```python
from build123d import *

# Parameters (mm, degrees)
SKETCH1_W                = 48
SKETCH1_H                = 20
BOSS_EXTRUDE1_DEPTH      = 300
BOSS_EXTRUDE2_DEPTH      = 24
BOSS_EXTRUDE2_DEPTH_BACK = 24
SKETCH2_R                = 20
BOSS_EXTRUDE3_DEPTH      = 24
BOSS_EXTRUDE3_DEPTH_BACK = 24
SKETCH3_R                = 20
CUT_EXTRUDE1_DEPTH       = 50
CUT_EXTRUDE1_DEPTH_BACK  = 50
SKETCH4_R                = 10
CUT_EXTRUDE2_DEPTH       = 50
CUT_EXTRUDE2_DEPTH_BACK  = 50
SKETCH5_R                = 10


with BuildPart() as part:
    # Sketch1 → Boss-Extrude1 (new body)
    with BuildSketch(Plane(origin=(0, 0, 0), x_dir=(0, 0, -1), z_dir=(1, 0, 0))):
        Rectangle(SKETCH1_W, SKETCH1_H)
    extrude(amount=BOSS_EXTRUDE1_DEPTH)

    # Sketch2 → Boss-Extrude2 (add, two sides: drawn at the far end of the back side and taken through both)
    with BuildSketch(Plane(origin=(0, 0, 0), x_dir=(1, 0, 0), z_dir=(0, 1, 0)).offset(-BOSS_EXTRUDE2_DEPTH_BACK)):
        with Locations(Location((0, 0, 0), (0, 0, 270))):
            Circle(SKETCH2_R)
    extrude(amount=BOSS_EXTRUDE2_DEPTH + BOSS_EXTRUDE2_DEPTH_BACK)

    # Sketch3 → Boss-Extrude3 (add, two sides: drawn at the far end of the back side and taken through both)
    with BuildSketch(Plane(origin=(0, 0, 0), x_dir=(1, 0, 0), z_dir=(0, 1, 0)).offset(-BOSS_EXTRUDE3_DEPTH_BACK)):
        with Locations(Location((300, 0, 0), (0, 0, 270))):
            Circle(SKETCH3_R)
    extrude(amount=BOSS_EXTRUDE3_DEPTH + BOSS_EXTRUDE3_DEPTH_BACK)

    # Sketch4 → Cut-Extrude1 (cut, two sides: drawn at the far end of the back side and taken through both)
    with BuildSketch(Plane(origin=(0, 0, 0), x_dir=(1, 0, 0), z_dir=(0, 1, 0)).offset(-CUT_EXTRUDE1_DEPTH_BACK)):
        with Locations(Location((0, 0, 0), (0, 0, 270))):
            Circle(SKETCH4_R)
    extrude(amount=CUT_EXTRUDE1_DEPTH + CUT_EXTRUDE1_DEPTH_BACK, mode=Mode.SUBTRACT)

    # Sketch5 → Cut-Extrude2 (cut, two sides: drawn at the far end of the back side and taken through both)
    with BuildSketch(Plane(origin=(0, 0, 0), x_dir=(1, 0, 0), z_dir=(0, 1, 0)).offset(-CUT_EXTRUDE2_DEPTH_BACK)):
        with Locations(Location((300, 0, 0), (0, 0, 270))):
            Circle(SKETCH5_R)
    extrude(amount=CUT_EXTRUDE2_DEPTH + CUT_EXTRUDE2_DEPTH_BACK, mode=Mode.SUBTRACT)


solid = part.part
```
CAD build for the part. Positions are in the model's coordinates, mm. A direction names the side the tool comes from. Give positions to 0.01 mm unless a question says otherwise; leave off trailing zeros. Loops run counter-clockwise (first coordinate to the right, second up) from the corner with the lowest first, then second, coordinate; pieces in that order, holes last. Notation, with made-up numbers: M 69,-33.5 L 111,-33.5 A25 cw 111,-5.5 Z; hole C -30.5,-31.5 d8. An arc over 180 degrees is marked long. Use one line per item in the form item = value.
Item 1: Which spindle directions (+Z, -Z, +X, -X, +Y, -Y) get a long thin tool onto all of the face, cutting with end or side? Do faces 4 (the face through (291.128, -0.336, 4.614)), 5 (the face through (319.83, -0.34, -2.6)). Say none if no direction does.
Determined:
face_4 = +Y, -Y
face_5 = none
Item 2: Two-plate mould, pull along X, no slides. Class faces 1 (the face through (148, -10, 0)), 2 (the face through (-19.524, -0.336, -4.336)), 3 (the face through (148, 0, -24)): pulls with the +X half, pulls with the -X half, needs draft (parallel to the pull), parting line crosses it, or undercut.
Determined:
face_1 = undercut
face_2 = undercut
face_3 = needs draft
Item 3: Drill centre lines: probe 1 along X at (y, z) = (2, 0); probe 2 along X at (y, z) = (14, 0); probe 3 along X at (y, z) = (8, -8). Where is each one in solid material? Low to high. Write a range as from..to.
Determined:
probe_1 = -20..-10, 10..290, 310..320
probe_2 = -20..-10, 10..20, 280..290, 310..320
probe_3 = -18.33..-6, 6..294, 306..318.33
Item 4: Flat gauge pins, fed straight in: pin 1 (12 mm diameter, centred on x = 96.5, z = -5.5, fed in from +Y); pin 2 (4.5 mm diameter, centred on y = 4.5, z = 22.5, fed in from -X); pin 3 (24 mm diameter, centred on x = 92, z = 7, fed in from -Y); pin 4 (12 mm diameter, centred on x = 300, z = 0, fed in from -Y). Where does each tip first touch, or does it go through?
Determined:
pin_1 = 10
pin_2 = 0
pin_3 = -10
pin_4 = through
Item 5: Slice it at D-D (x = 204). List the corners of the cut face in (y, z), plus the area to 3 significant figures.
Determined:
outline = M -10,-24 L 10,-24 L 10,24 L -10,24 Z
area = 960 mm2
Item 6: Slice it at B-B (z = 0). List the corners of the cut face in (x, y).
Determined:
outline = M -20,-24 L -10,-24 L -10,24 L -20,24 Z; M 10,-24 L 20,-24 L 20,-10 L 280,-10 L 280,-24 L 290,-24 L 290,24 L 280,24 L 280,10 L 20,10 L 20,24 L 10,24 Z; M 310,-24 L 320,-24 L 320,24 L 310,24 Z
Item 7: Slice it at A-A (y = -1). List the corners of the cut face in (x, z).
Determined:
outline = M 0,-24 L 300,-24 L 300,-20 A20 ccw 300,20 L 300,24 L 0,24 L 0,20 A20 ccw 0,-20 Z; hole C 0,0 d20; hole C 300,0 d20
Item 8: Slice it at C-C (y = 20.5). List the corners of the cut face in (x, z), plus the area to 3 significant figures.
Determined:
outline = C 0,0 d40; C 300,0 d40; hole C 0,0 d20; hole C 300,0 d20
area = 1,880 mm2
